from build123d import *

# Parameters (mm, degrees)
BOSS_EXTRUDE1_DEPTH = 5
SKETCH3_R           = 10
CUT_EXTRUDE1_DEPTH  = 5


with BuildPart() as part:
    # Sketch2 → Boss-Extrude1 (new body)
    with BuildSketch(Plane.XY):
        Polygon((-26.751257452, 29.870014622), (-11.751257452, 29.870014622), (-11.751257452, 34.870014622), (8.248742548, 34.870014622), (8.248742548, 29.870014622), (23.248742548, 29.870014622), (23.248742548, 14.870014622), (28.248742548, 14.870014622), (28.248742548, -5.129985378), (23.248742548, -5.129985378), (23.248742548, -20.129985378), (-26.751257452, -20.129985378), (-26.751257452, -5.129985378), (-31.751257452, -5.129985378), (-31.751257452, 14.870014622), (-26.751257452, 14.870014622), align=None)
    extrude(amount=BOSS_EXTRUDE1_DEPTH)

    # Sketch3 → Cut-Extrude1 (cut)
    with BuildSketch(Plane.XY.offset(5)):
        with Locations((-1.751257452, 8.827972436)):
            Circle(SKETCH3_R)
        Polygon((-3.751257452, -20.129985378), (-3.751257452, -14.129985378), (-5.251257452, -14.129985378), (-5.251257452, -10.129985378), (-3.751257452, -10.129985378), (-3.751257452, -8.129985378), (0.248742548, -8.129985378), (0.248742548, -10.129985378), (1.748742548, -10.129985378), (1.748742548, -14.129985378), (0.248742548, -14.129985378), (0.248742548, -20.129985378), align=None)
    extrude(amount=-CUT_EXTRUDE1_DEPTH, mode=Mode.SUBTRACT)


solid = part.part
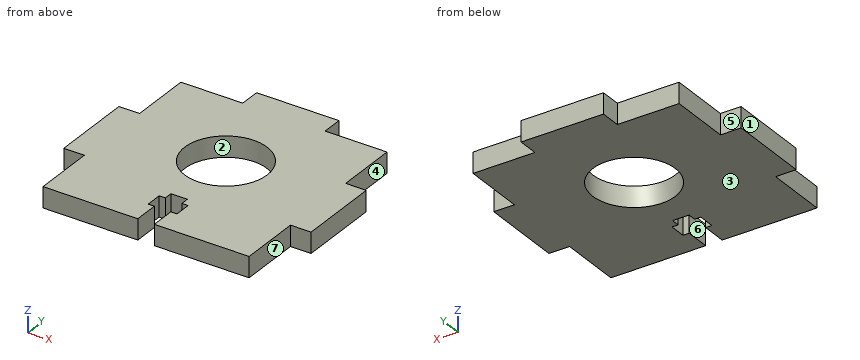
Geometry: final body of the model. Coordinates: model frame, mm. Face numbers are marked on the shaded views. A direction names the side the tool comes from. Round coordinates to 2 decimals unless told otherwise and drop trailing zeros. Loops run counter-clockwise (first coordinate to the right, second up) from the corner with the lowest first, then second, coordinate; pieces in that order, holes last. Notation, with made-up numbers: M 3.5,87.25 L 36.5,87.25 A28 ccw 36.5,115.25 Z; hole C -2,11 d4. An arc over 180 degrees is marked long. Put each result on its own line as item: value. Start each with the question number.
(1) Draft query along X for the marked faces 1, 2 and 3. Return one class per face: +X half, -X half, draft (parallel to the pull), parting line (faces both ways), or undercut.
(2) Set-up query: the marked faces 4, 5, 6 and 7. Return all of +Z, -Z, +X, -X, +Y, -Y with unobstructed straight access to the full face (end or side cutting, diameter ignored); none if empty.
(3) Material intervals for line 1 along X through (y, z) = (-9.5, 3.6); line 2 along X through (y, z) = (-10.5, 0.55); line 3 along Y through (x, z) = (-14, 4.85), sorted ascending. Write a range as [from, to].
(4) Contact query for flat-ended pins moving along their axis: pin 1 Ø2.5 at (y, z) = (-15, 2.5) entering from +X; pin 2 Ø1 at (y, z) = (-9, 3) entering from -X; pin 3 Ø1.5 at (y, z) = (31.5, 3) entering from +X. Output: stop coordinate, or through.
(5) Section query A-A (y = 2). Return loops of the section in (x, z), then the cut area to 3 significant figures.
(6) Section query C-C (x = -19). Return loops of the section in (y, z), then the cut area to 3 significant figures.
(7) Section query D-D (y = 14). Return loops of the section in (x, z), then the cut area to 3 significant figures.
Findings below:
1. face 1: -X half
1. face 2: undercut
1. face 3: draft
2. face 4: +Z, -Z, +X, +Y
2. face 5: +Z, -Z, -X, +Y
2. face 6: +Z, -Z, -Y
2. face 7: +Z, -Z, +X, -Y
3. line 1: x = [-26.75, -3.75], [0.25, 23.25]
3. line 2: x = [-26.75, -5.25], [1.75, 23.25]
3. line 3: y = [-20.13, 29.87]
4. pin 1: stops at x = 23.25
4. pin 2: stops at x = -26.75
4. pin 3: stops at x = 8.25
5. outline: M -31.75,0 L -9.06,0 L -9.06,5 L -31.75,5 Z; M 5.55,0 L 28.25,0 L 28.25,5 L 5.55,5 Z
5. area: 227 mm2
6. outline: M -20.13,0 L 29.87,0 L 29.87,5 L -20.13,5 Z
6. area: 250 mm2
7. outline: M -31.75,0 L -10.31,0 L -10.31,5 L -31.75,5 Z; M 6.81,0 L 28.25,0 L 28.25,5 L 6.81,5 Z
7. area: 214 mm2
